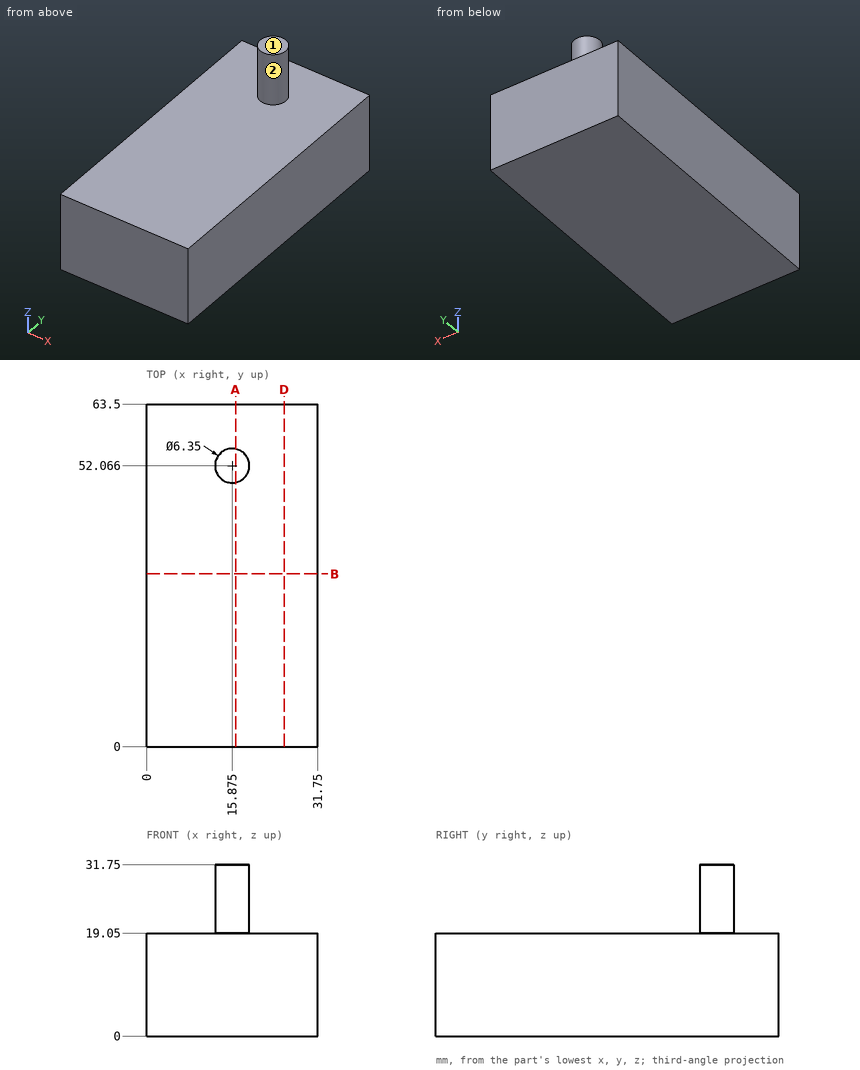
Geometry: see drawing. Coordinates: mm, zero at the bounding-box minimum. A direction names the side the tool comes from. Coordinates: 2 decimals unless noted, no trailing zeros. Loops run counter-clockwise (first coordinate to the right, second up) from the corner with the lowest first, then second, coordinate; pieces in that order, holes last. Notation, with made-up numbers: (-34.5, 19.5) -> (-27.5, 19.5) arc R32 cw to (-27.5, 56.5) -> close; hole circle Ø5 at (-34.75, 11). An arc over 180 degrees is marked (long way). Write item = value, one per line. Start each with the question number.
Item 1: Material intervals for line 1 (Z direction, x = 28, y = 39), sorted ascending.
Item 2: Reachability of the marked faces 1 and 2 from +Z, -Z, +X, -X, +Y, -Y: full face, straight path, thin tool, end or side. Return the list, or none.
Item 3: Cut plane A-A, the plane x = 16.5. Return loops of the section in (y, z).
Item 4: Cut plane D-D, the plane x = 25.5. Return loops of the section in (y, z).
Item 5: First-contact query: P1, Ø3, axis at x = 16, y = 16.5, coming from the +Z side. Flat tip, straight axial feed; report the tip coordinate or a pass-through.
Item 6: Cut plane B-B, the plane y = 32. Return loops of the section in (x, z).
Ans:
q1.line_1 = 0 to 19.05
q2.face_1 = +Z, +X, -X, +Y, -Y
q2.face_2 = +Z
q3.outline = (0, 0) -> (63.5, 0) -> (63.5, 19.05) -> (55.18, 19.05) -> (55.18, 31.75) -> (48.95, 31.75) -> (48.95, 19.05) -> (0, 19.05) -> close
q4.outline = (0, 0) -> (63.5, 0) -> (63.5, 19.05) -> (0, 19.05) -> close
q5.P1 = 19.05
q6.outline = (0, 0) -> (31.75, 0) -> (31.75, 19.05) -> (0, 19.05) -> close
